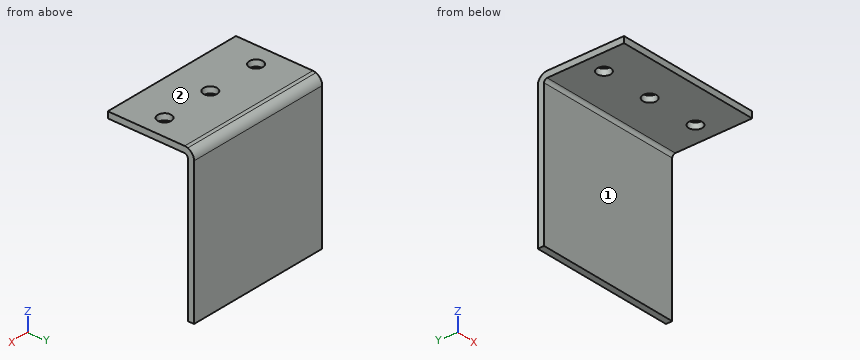
```python
from build123d import *

# Parameters (mm, degrees)
SKETCH_1_W             = 110
SKETCH_1_H             = 3
SM_BASE_FLANGE_1_DEPTH = 35
OTHER_START            = -35
OTHER_1_DEPTH          = 70
OTHER_1_2_DEPTH        = 70
SKETCH_9_R             = 3.25
CUT_EXTRUDE_3_DEPTH    = 90.55412418


# Read off the part's stored shape, not the designer's step: Нарисованный сгиб1
# Sheet-metal steps are written as plain solids
with BuildPart() as part:
    # Sketch 1 → Базовая кромка1 (new, symmetric)
    with BuildSketch(Plane(origin=(0, 0, 0), x_dir=(0, 0, -1), z_dir=(1, 0, 0))):
        with Locations((15, 1.5)):
            Rectangle(SKETCH_1_W, SKETCH_1_H)
    extrude(amount=SM_BASE_FLANGE_1_DEPTH, both=True)

    # Other 1 outline → Other 1 (cut)
    with BuildSketch(Plane.YZ.offset(OTHER_START)):
        with BuildLine():
            Line((0, 40), (0, 2.742640687))
            ThreePointArc((0, 2.742640687), (2.174234614, 1.098076211), (3, -1.5))
            Line((3, -1.5), (3, 40))
            Line((3, 40), (0, 40))
        make_face()
    extrude(amount=OTHER_1_DEPTH, mode=Mode.SUBTRACT)

    # Other 1 2 outline → Other 1 2 (add)
    with BuildSketch(Plane.YZ.offset(OTHER_START)):
        with BuildLine():
            Line((-1.5, 3), (-38.28761102, 3))
            Line((-38.28761102, 3), (-38.28761102, 0))
            Line((-38.28761102, 0), (-1.5, 0))
            ThreePointArc((-1.5, 0), (-0.439339828, -0.439339828), (0, -1.5))
            Line((0, -1.5), (0, 2.742640687))
            ThreePointArc((0, 2.742640687), (-0.739041096, 2.935193518), (-1.5, 3))
        make_face()
    extrude(amount=OTHER_1_2_DEPTH)

    # Эскиз9 → Вырез-Вытянуть3 (cut, through all)
    with BuildSketch(Plane.XY.offset(3)):
        with Locations((-25, -19.89380551)):
            Circle(SKETCH_9_R)
        with Locations((0, -19.89380551)):
            Circle(SKETCH_9_R)
        with Locations((25, -19.89380551)):
            Circle(SKETCH_9_R)
    extrude(amount=-CUT_EXTRUDE_3_DEPTH, mode=Mode.SUBTRACT)


solid = part.part
```
Part model, mm, in its own coordinate system. Face numbers are marked on the shaded views. A direction names the side the tool comes from. Round coordinates to 2 decimals unless told otherwise and drop trailing zeros. Write each loop counter-clockwise with the first axis right and the second up, starting at its lowest first coordinate (ties: lowest second). Pieces come first, ordered by that corner, then holes.
Item 1: Cut at B-B, the plane x = -7. Give the cut face in (y, z).
Results:
outline: (-38.29, 0) - (-1.5, 0) arc R1.5 cw to (0, -1.5) - (0, -70) - (3, -70) - (3, -1.5) arc R4.5 ccw to (-1.5, 3) - (-38.29, 3) - close
Item 2: Cut at A-A, the plane x = 25. Give the cut face in (y, z), plus the area to 4 significant figures.
Results:
outline: (-38.29, 0) - (-23.14, 0) - (-23.14, 3) - (-38.29, 3) - close; (-16.64, 0) - (-1.5, 0) arc R1.5 cw to (0, -1.5) - (0, -70) - (3, -70) - (3, -1.5) arc R4.5 ccw to (-1.5, 3) - (-16.64, 3) - close
area: 310.5 mm2
Item 3: Probe L1, parallel to Z at x = -11.5, y = -6; L2, parallel to Y at x = 25, z = 0.85. List the from-to ranges inside material, lowest first.
Results:
L1: z = 0 to 3
L2: y = -38.29 to -23.14, -16.64 to 2.34
Item 4: Which spindle directions (+Z, -Z, +X, -X, +Y, -Y) get a long thin tool onto all of the face, cutting with end or side? Do the marked faces 1 and 2. Say none if no direction does.
Results:
face 1: -Z, +X, -X, -Y
face 2: +Z, +X, -X, +Y, -Y
Item 5: Drop flat-ended pins along their axis: pin 1 Ø20.5 at (x, z) = (-4, -49) entering from -Y; pin 2 Ø7.5 at (x, y) = (25, -19.89) entering from -Z; pin 3 Ø8.5 at (x, y) = (0, -19.89) entering from +Z. Give the stop position or say it passes through.
Results:
pin 1: stops at y = 0
pin 2: stops at z = 0
pin 3: stops at z = 3
Item 6: Cut at C-C, the plane y = -9. Give the cut face in (x, z).
Results:
outline: (-35, 0) - (35, 0) - (35, 3) - (-35, 3) - close
